```python
from build123d import *

# Parameters (mm, degrees)
SKETCH_1_W          = 40
SKETCH_1_H          = 20
EXTRUDE_1_DEPTH     = 3
SKETCH_2_W          = 40
SKETCH_2_H          = 4
EXTRUDE_2_DEPTH     = 44.5
SKETCH_3_R          = 10
SKETCH_3_R_2        = 2
CUT_EXTRUDE_1_DEPTH = 54.965266607
FILLET_1_R          = 20
SKETCH_4_W          = 3
SKETCH_4_H          = 16
EXTRUDE_3_DEPTH     = 15
CUT_EXTRUDE_2_DEPTH = 63.898728127
FILLET_2_R          = 5
FILLET_3_R          = 3
SKETCH_6_R          = 1.5
CUT_EXTRUDE_3_DEPTH = 3
SKETCH_7_R          = 2
CUT_EXTRUDE_4_DEPTH = 54.965266607


with BuildPart() as part:
    # 草图1 → 凸台-拉伸1 (new body)
    with BuildSketch(Plane(origin=(0, 0, 0), x_dir=(1, 0, 0), z_dir=(0, 1, 0))):
        Rectangle(SKETCH_1_W, SKETCH_1_H)
    extrude(amount=EXTRUDE_1_DEPTH)

    # 草图2 → 凸台-拉伸2 (add)
    with BuildSketch(Plane(origin=(0, 3, 0), x_dir=(1, 0, 0), z_dir=(0, 1, 0))):
        with Locations((0, 8)):
            Rectangle(SKETCH_2_W, SKETCH_2_H)
    extrude(amount=EXTRUDE_2_DEPTH)

    # 草图3 → 切除-拉伸1 (cut, through all)
    with BuildSketch(Plane.XY.offset(-6)):
        with Locations((0, 24)):
            Circle(SKETCH_3_R)
        with Locations((12.727922061, 36.727922061)):
            Circle(SKETCH_3_R_2)
        with Locations((12.727922061, 11.272077939)):
            Circle(SKETCH_3_R_2)
        with Locations((-12.727922061, 11.272077939)):
            Circle(SKETCH_3_R_2)
        with Locations((-12.727922061, 36.727922061)):
            Circle(SKETCH_3_R_2)
    extrude(amount=-CUT_EXTRUDE_1_DEPTH, mode=Mode.SUBTRACT)

    # 圆角1
    fillet_1_edges = [part.edges().sort_by_distance(p)[0] for p in [
        (20, 47.5, -8),
        (-20, 47.5, -8),
    ]]
    fillet(fillet_1_edges, radius=FILLET_1_R - 0.0001)  # a hair under: the kernel refuses the full size

    # 草图4 → 凸台-拉伸3 (add)
    with BuildSketch(Plane(origin=(0, 3, 0), x_dir=(1, 0, 0), z_dir=(0, 1, 0))):
        with Locations((-18.5, -2)):
            Rectangle(SKETCH_4_W, SKETCH_4_H)
        with Locations((18.5, -2)):
            Rectangle(SKETCH_4_W, SKETCH_4_H)
    extrude(amount=EXTRUDE_3_DEPTH)

    # 草图5 → 切除-拉伸2 (cut, through all)
    with BuildSketch(Plane.ZY.offset(20)):
        Polygon((-6, 18), (10, 3), (10, 18), align=None)
    extrude(amount=-CUT_EXTRUDE_2_DEPTH, mode=Mode.SUBTRACT)

    # 圆角2
    fillet_2_edges = [part.edges().sort_by_distance(p)[0] for p in [
        (-18.5, 18, -6),
        (18.5, 18, -6),
    ]]
    fillet(fillet_2_edges, radius=FILLET_2_R)

    # 圆角3
    fillet_3_edges = [part.edges().sort_by_distance(p)[0] for p in [
        (-17, 3, 2),
        (17, 3, 2),
    ]]
    fillet(fillet_3_edges, radius=FILLET_3_R)

    # 草图6 → 切除-拉伸3 (cut)
    with BuildSketch(Plane(origin=(0, 3, 0), x_dir=(1, 0, 0), z_dir=(0, 1, 0))):
        with Locations(Location((-9, 2, 0), (0, 0, 270))):
            Circle(SKETCH_6_R)
        with Locations(Location((9, 2, 0), (0, 0, 90))):
            Circle(SKETCH_6_R)
        with Locations(Location((9, -6, 0), (0, 0, 270))):
            Circle(SKETCH_6_R)
        with Locations(Location((-9, -6, 0), (0, 0, 90))):
            Circle(SKETCH_6_R)
    extrude(amount=-CUT_EXTRUDE_3_DEPTH, mode=Mode.SUBTRACT)

    # 草图7 → 切除-拉伸4 (cut, through all)
    with BuildSketch(Plane.XY.offset(-6)):
        with Locations((0, 40)):
            Circle(SKETCH_7_R)
        with Locations((-16, 24)):
            Circle(SKETCH_7_R)
        with Locations((0, 8)):
            Circle(SKETCH_7_R)
        with Locations((16, 24)):
            Circle(SKETCH_7_R)
    extrude(amount=-CUT_EXTRUDE_4_DEPTH, mode=Mode.SUBTRACT)


solid = part.part
```
The listing builds one solid part. Answer for the finished solid, in the listing's coordinates (mm). A direction names the side the tool comes from. Coordinates: 2 decimals unless noted, no trailing zeros. Write each loop counter-clockwise with the first axis right and the second up, starting at its lowest first coordinate (ties: lowest second). Pieces come first, ordered by that corner, then holes. Notation, with made-up numbers: M 81.25,5 L 137.25,5 A17 ccw 137.25,36 Z; hole C 3,-2.75 d5. An arc over 180 degrees is marked long. Use a Markdown table: item, result. Add a question column.
1. For a pull along X with two mould halves and no side action, classify faces 1 (the cylindrical face through (-16.1, 3.86, 1.89)), 2 (the cylindrical face through (-11.8, 9.5, -8)), 3 (the cylindrical face through (13.986, 41.797, -8.028)), 4 (the flat face through (0, 0, 0)) as +X half, -X half, draft (parallel to the pull), parting line (faces both ways), or undercut.
2. Section D-D (y = 40) is taken. Give the vertices of the cut face in (x, z).
3. Which of the six approach directions +Z, -Z, +X, -X, +Y, -Y give full straight-line access (tool end or side, diameter ignored) to faces 5 (the flat face through (17, 10, -2)), 6 (the cylindrical face through (-1.302, 33.915, -7.972))?
4. Straight lines are drawn through the part: line 1 along X through (y, z) = (1.1, -2); line 2 along Y through (x, z) = (12, -7.75); line 3 along Z through (x, y) = (-15, 36). For each, find the intervals that lie inside material, in ascending order. Write a range as [from, to].
5. Section B-B (x = 3) is taken. Give the vertices of the cut face in (y, z).
6. Given P1, Ø10, axis at x = -3.5, z = 2, coming from the +Y side; P2, Ø12, axis at x = 9.5, y = 27, coming from the +Z side; P3, Ø1.8, axis at x = 9, z = 6, coming from the +Y side; P4, Ø6, axis at y = 36.5, z = -4, coming from the +X side, each flat-ended and moving along its own axis, determine where each tip first touches the part or whether it passes through.
7. Section C-C (z = 2) is taken. Give the vertices of the cut face in (x, y), plus the area to 3 significant figures.
8. Section A-A (y = 24) is taken. Give the vertices of the cut face in (x, z).
Data:
| question | item | result |
|---|---|---|
| 1 | face 1 | undercut |
| 1 | face 2 | undercut |
| 1 | face 3 | +X half |
| 1 | face 4 | draft |
| 2 | outline | M -15.61,-10 L -2,-10 L -2,-6 L -15.61,-6 Z; M 2,-10 L 15.61,-10 L 15.61,-6 L 2,-6 Z |
| 3 | face 5 | +Z, +Y |
| 3 | face 6 | +Z, -Z |
| 4 | line 1 | x = [-20, -10.5], [-7.5, 7.5], [10.5, 20] |
| 4 | line 2 | y = [0, 9.41], [13.13, 34.87], [38.59, 43.5] |
| 4 | line 3 | z = [-10, -6] |
| 5 | outline | M 0,-10 L 14.46,-10 L 14.46,-6 L 3,-6 L 3,10 L 0,10 Z; M 33.54,-10 L 47.27,-10 L 47.27,-6 L 33.54,-6 Z |
| 6 | P1 | stops at y = 3 |
| 6 | P2 | stops at z = -6 |
| 6 | P3 | passes through |
| 6 | P4 | stops at x = 18.82 |
| 7 | outline | M -20,0 L 20,0 L 20,10.5 L 17,10.5 L 17,6 A3 cw 14,3 L -14,3 A3 cw -17,6 L -17,10.5 L -20,10.5 Z |
| 7 | area | 169 mm2 |
| 8 | outline | M -20,-10 L -18,-10 L -18,-6 L -20,-6 Z; M -14,-10 L -10,-10 L -10,-6 L -14,-6 Z; M 10,-10 L 14,-10 L 14,-6 L 10,-6 Z; M 18,-10 L 20,-10 L 20,-6 L 18,-6 Z |
